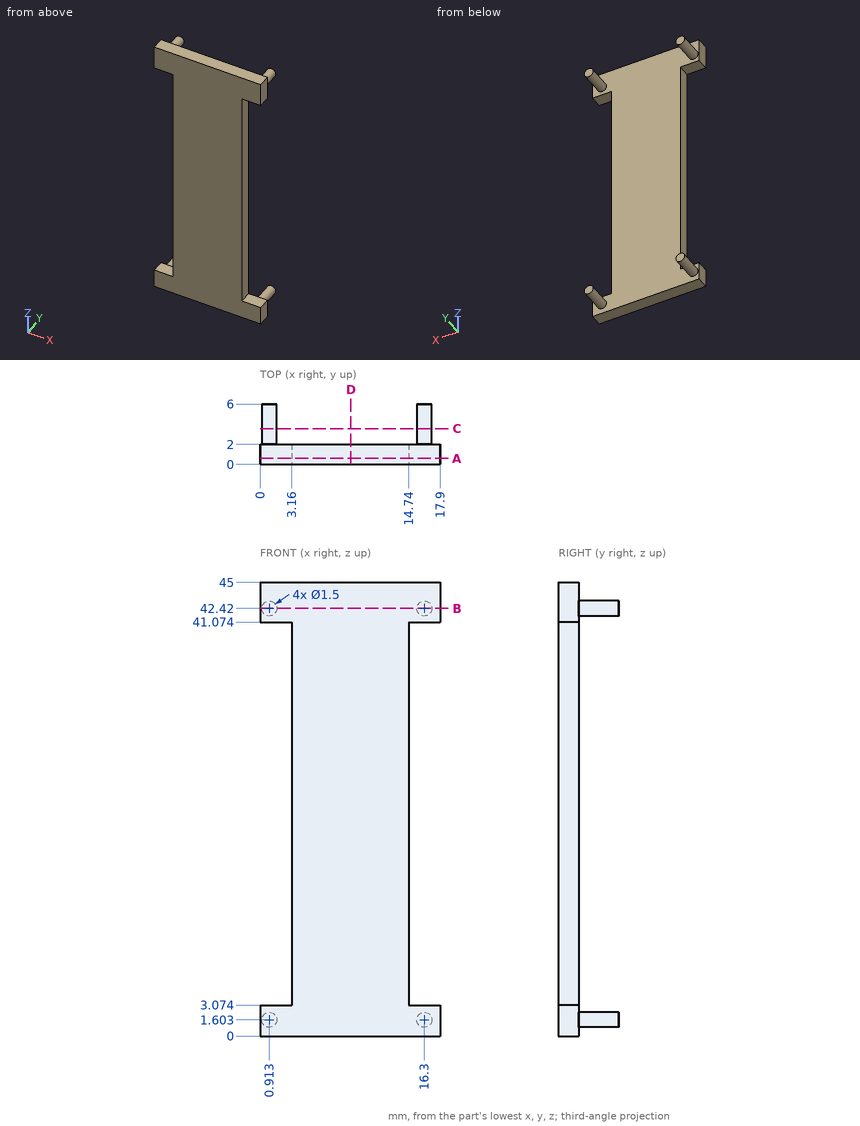
Geometry: see drawing. Coordinates: mm, zero at the bounding-box minimum. Give positions to 0.01 mm unless a question says otherwise; leave off trailing zeros. Order: outer loops, then holes, each group sorted by start corner. A loop starts at its lowest first (then second) coordinate and runs counter-clockwise, first axis right, second up. Notation, with made-up numbers: (58, 28) - (89, 28) arc R18 ccw to (89, 53) - close; hole circle Ø10 at (85, 5). An arc over 180 degrees is marked (long way). Use a Markdown table: item, result.
(1) Section query A-A (y = 0.6). Output: boundary loops of the cut face in (x, z) (1 decimal), then the cut area to 3 significant figures.
Computed values:
| item | result |
|---|---|
| outline | (0, 0) - (17.9, 0) - (17.9, 3.1) - (14.7, 3.1) - (14.7, 41.1) - (17.9, 41.1) - (17.9, 45) - (0, 45) - (0, 41.1) - (3.2, 41.1) - (3.2, 3.1) - (0, 3.1) - close |
| area | 565 mm2 |
(2) Section query C-C (y = 3.55). Output: boundary loops of the cut face in (x, z).
Computed values:
| item | result |
|---|---|
| outline | circle Ø1.5 at (0.91, 1.6); circle Ø1.5 at (0.91, 42.42); circle Ø1.5 at (16.3, 1.6); circle Ø1.5 at (16.3, 42.42) |
(3) Pin query (flat end, axial travel): pin 1 (1.5 mm diameter, centred on x = 3.5, y = 3.5, fed in from -Z); pin 2 (0.6 mm diameter, centred on y = 1, z = 18.5, fed in from -X); pin 3 (1 mm diameter, centred on y = 1.5, z = 14, fed in from +X). Return the tip coordinate at first contact, or that it passes through.
Computed values:
| item | result |
|---|---|
| pin 1 | passes through |
| pin 2 | stops at x = 3.16 |
| pin 3 | stops at x = 14.74 |
(4) Line query: line 1 (Z direction, x = 1.5, y = 1.45) (1 decimal); line 2 (Y direction, x = 13.5, z = 14); line 3 (X direction, y = 0.9, z = 26). Output: solid intervals per line, ascending. Write a range as from..to.
Computed values:
| item | result |
|---|---|
| line 1 | z = 0..3.1, 41.1..45 |
| line 2 | y = 0..2 |
| line 3 | x = 3.16..14.74 |
(5) Section query D-D (x = 9). Output: boundary loops of the cut face in (y, z).
Computed values:
| item | result |
|---|---|
| outline | (0, 0) - (2, 0) - (2, 45) - (0, 45) - close |
(6) Section query B-B (z = 42.42). Output: boundary loops of the cut face in (x, y).
Computed values:
| item | result |
|---|---|
| outline | (0, 0) - (17.9, 0) - (17.9, 2) - (17.05, 2) - (17.05, 6) - (15.55, 6) - (15.55, 2) - (1.66, 2) - (1.66, 6) - (0.16, 6) - (0.16, 2) - (0, 2) - close |
